Here's how the part is built. I have some questions about the finished solid (model axes, mm). A direction names the side the tool comes from. Round coordinates to 2 decimals unless told otherwise and drop trailing zeros. One line per question, with ' | ' between items. Start each with the question number.
```python
from build123d import *

# Parameters (mm, degrees)
SKETCH1_W           = 633
SKETCH1_H           = 333
BOSS_EXTRUDE1_DEPTH = 12
CUT_EXTRUDE1_DEPTH  = 13


with BuildPart() as part:
    # Sketch1 → Boss-Extrude1 (new body)
    with BuildSketch(Plane(origin=(0, 0, 0), x_dir=(1, 0, 0), z_dir=(0, 1, 0))):
        Rectangle(SKETCH1_W, SKETCH1_H)
    extrude(amount=BOSS_EXTRUDE1_DEPTH)

    # Sketch2 → Cut-Extrude1 (cut, through all)
    with BuildSketch(Plane(origin=(0, 12, 0), x_dir=(1, 0, 0), z_dir=(0, 1, 0))):
        with BuildLine():
            Line((-227.75, -164.5), (-214.25, -164.5))
            ThreePointArc((-214.25, -164.5), (-212.835786438, -165.085786438), (-212.25, -166.5))
            Line((-212.25, -166.5), (-212.25, -168.5))
            Line((-212.25, -168.5), (-229.75, -168.5))
            Line((-229.75, -168.5), (-229.75, -166.5))
            ThreePointArc((-229.75, -166.5), (-229.164213562, -165.085786438), (-227.75, -164.5))
        make_face()
        with BuildLine():
            Line((316.5, -62.25), (318.5, -62.25))
            Line((318.5, -62.25), (318.5, -79.75))
            Line((318.5, -79.75), (316.5, -79.75))
            ThreePointArc((316.5, -79.75), (315.085786438, -79.164213562), (314.5, -77.75))
            Line((314.5, -77.75), (314.5, -64.25))
            ThreePointArc((314.5, -64.25), (315.085786438, -62.835786438), (316.5, -62.25))
        make_face()
        with BuildLine():
            Line((212.25, -166.5), (212.25, -168.5))
            Line((212.25, -168.5), (229.75, -168.5))
            Line((229.75, -168.5), (229.75, -166.5))
            ThreePointArc((229.75, -166.5), (229.164213562, -165.085786438), (227.75, -164.5))
            Line((227.75, -164.5), (214.25, -164.5))
            ThreePointArc((214.25, -164.5), (212.835786438, -165.085786438), (212.25, -166.5))
        make_face()
        with BuildLine():
            Line((318.5, 62.25), (318.5, 79.75))
            Line((318.5, 79.75), (316.5, 79.75))
            ThreePointArc((316.5, 79.75), (315.085786438, 79.164213562), (314.5, 77.75))
            Line((314.5, 77.75), (314.5, 64.25))
            ThreePointArc((314.5, 64.25), (315.085786438, 62.835786438), (316.5, 62.25))
            Line((316.5, 62.25), (318.5, 62.25))
        make_face()
        with BuildLine():
            Line((-316.5, 62.25), (-318.5, 62.25))
            Line((-318.5, 62.25), (-318.5, 79.75))
            Line((-318.5, 79.75), (-316.5, 79.75))
            ThreePointArc((-316.5, 79.75), (-315.085786438, 79.164213562), (-314.5, 77.75))
            Line((-314.5, 77.75), (-314.5, 64.25))
            ThreePointArc((-314.5, 64.25), (-315.085786438, 62.835786438), (-316.5, 62.25))
        make_face()
        with BuildLine():
            Line((-318.5, -62.25), (-318.5, -79.75))
            Line((-318.5, -79.75), (-316.5, -79.75))
            ThreePointArc((-316.5, -79.75), (-315.085786438, -79.164213562), (-314.5, -77.75))
            Line((-314.5, -77.75), (-314.5, -64.25))
            ThreePointArc((-314.5, -64.25), (-315.085786438, -62.835786438), (-316.5, -62.25))
            Line((-316.5, -62.25), (-318.5, -62.25))
        make_face()
        with BuildLine():
            Line((227.75, 164.5), (214.25, 164.5))
            ThreePointArc((214.25, 164.5), (212.835786438, 165.085786438), (212.25, 166.5))
            Line((212.25, 166.5), (212.25, 168.5))
            Line((212.25, 168.5), (229.75, 168.5))
            Line((229.75, 168.5), (229.75, 166.5))
            ThreePointArc((229.75, 166.5), (229.164213562, 165.085786438), (227.75, 164.5))
        make_face()
        with BuildLine():
            Line((-212.25, 166.5), (-212.25, 168.5))
            Line((-212.25, 168.5), (-229.75, 168.5))
            Line((-229.75, 168.5), (-229.75, 166.5))
            ThreePointArc((-229.75, 166.5), (-229.164213562, 165.085786438), (-227.75, 164.5))
            Line((-227.75, 164.5), (-214.25, 164.5))
            ThreePointArc((-214.25, 164.5), (-212.835786438, 165.085786438), (-212.25, 166.5))
        make_face()
    extrude(amount=-CUT_EXTRUDE1_DEPTH, mode=Mode.SUBTRACT)


solid = part.part
```
1) I'm going to push flat-ended pins straight in: pin 1 Ø6 at (y, z) = (9, 72.5) entering from -X; pin 2 Ø3.5 at (x, y) = (-218, 3.5) entering from -Z. Where does each tip first touch, or does it pass through?
2) We'd pull the mould along Z, two halves only. Please class faces 1 (the face through (316.5, 6, 1)), 2 (the face through (-3, 6, 166.5)), 3 (the face through (221, 6, -164.5)), 4 (the face through (-314.5, 6, 71)): pulls with the +Z half, pulls with the -Z half, needs draft (parallel to the pull), parting line crosses it, or undercut.
3) For faces 5 (the face through (-221, 6, -164.5)), 6 (the face through (314.5, 6, -71)), 7 (the face through (-221, 6, 164.5)), 8 (the face through (-314.5, 6, -71)), 9 (the face through (-274, 6, 166.5)), which set-ups out of +Z, -Z, +X, -X, +Y, -Y let a thin tool reach every point of the face, with its end or its side?
4) Please list where these lines run through material, in increasing order: L1, parallel to Z at x = -219, y = 1.75; L2, parallel to X at y = 4.25, z = 74. Write a range as from..to.
Results are:
1) pin 1: x = -314.5 | pin 2: z = -164.5
2) face 1: needs draft | face 2: pulls with the +Z half | face 3: pulls with the -Z half | face 4: undercut
3) face 5: -Z, +Y, -Y | face 6: +X, +Y, -Y | face 7: +Z, +Y, -Y | face 8: -X, +Y, -Y | face 9: +Z, +X, -X, +Y, -Y
4) L1: -164.5..164.5 | L2: -314.5..314.5
